Here's how the part is built. I have some questions about the finished solid (model axes, mm). A direction names the side the tool comes from. Give positions to 0.01 mm unless a question says otherwise; leave off trailing zeros. Loops run counter-clockwise (first coordinate to the right, second up) from the corner with the lowest first, then second, coordinate; pieces in that order, holes last.
Q1. We'd pull the mould along Y, two halves only. Please class faces 3 (the face through (0, 8, 4)), 4 (the face through (0, -8.5, 1)), 5 (the face through (8.5, 0, 1)), 6 (the face through (0, 2.1, 2)): +Y half, -Y half, draft (parallel to the pull), parting line (faces both ways), or undercut.
Q2. I need wall thicknesses on line 1 (Y direction, x = 3, z = 2.25); line 2 (X direction, y = -1.25, z = 1.5) (1 decimal); line 3 (X direction, y = 2, z = 2.75) (3 decimals). Which ranges of each line are inside material? Lowest first, please.
Q3. For faces 1 (the face through (0, -2.1, 2)), 2 (the face through (-8.5, 0, 1)), which set-ups out of +Z, -Z, +X, -X, +Y, -Y let a thin tool reach every point of the face, with its end or its side?
Q4. If we section it at D-D (z = 0.25): Please give me the cut outline in (x, y) (3 decimals), plus the area to 3 significant figures.
Q5. If we section it at B-B (y = 6): Please give me the cut outline in (x, z).
Q6. Will this pin go through, and if not, where does the flat tip stop? P1, Ø6.5, axis at x = 2.5, y = 2.5, coming from the -Z side.
Q7. If we section it at A-A (z = 2.25): Please give me the cut outline in (x, y) (3 decimals), plus the area to 3 significant figures.
from build123d import *
from OCP.BRepFilletAPI import BRepFilletAPI_MakeChamfer

# Parameters (mm, degrees)
SKETCH1_R           = 2.75
BOSS_EXTRUDE1_DEPTH = 4
SKETCH2_W           = 17
SKETCH2_H           = 17
BOSS_EXTRUDE2_DEPTH = 1
SKETCH3_W           = 17
SKETCH3_H           = 17
SKETCH3_W_2         = 15
SKETCH3_H_2         = 15
BOSS_EXTRUDE3_DEPTH = 6
CHAMFER1_SIZE       = 1.5
CHAMFER2_SIZE       = 4
CHAMFER2_SIZE2      = 0.5
CUT_EXTRUDE1_DEPTH  = 0.6
BOSS_EXTRUDE4_START = 0.5
SKETCH5_W           = 14.989533589
SKETCH5_H           = 15
SKETCH5_R           = 2.75
BOSS_EXTRUDE4_DEPTH = 0.5


with BuildPart() as part:
    # Sketch1 → Boss-Extrude1 (new body)
    with BuildSketch(Plane(origin=(0, 0, 0), x_dir=(0, 1, 0), z_dir=(0, 0, 1))):
        with Locations(Location((0, 0, 0), (0, 0, 270))):
            Circle(SKETCH1_R)
        Polygon((-0.7, -0.625), (-2.1, -0.625), (-2.1, 0.625), (-0.7, 0.625), (-0.7, 2.1), (0.7, 2.1), (0.7, 0.625), (2.1, 0.625), (2.1, -0.625), (0.7, -0.625), (0.7, -2.1), (-0.7, -2.1), align=None, mode=Mode.SUBTRACT)
    extrude(amount=BOSS_EXTRUDE1_DEPTH)

    # Sketch2 → Boss-Extrude2 (add)
    with BuildSketch(Plane.XY.offset(4)):
        Rectangle(SKETCH2_W, SKETCH2_H)
    extrude(amount=BOSS_EXTRUDE2_DEPTH)

    # Sketch3 → Boss-Extrude3 (add)
    with BuildSketch(Plane(origin=(0, 0, 4), x_dir=(1, 0, 0), z_dir=(0, 0, -1))):
        Rectangle(SKETCH3_W, SKETCH3_H)
        Rectangle(SKETCH3_W_2, SKETCH3_H_2, mode=Mode.SUBTRACT)
    extrude(amount=BOSS_EXTRUDE3_DEPTH)

    # Chamfer1
    chamfer1_edges = [part.edges().sort_by_distance(p)[0] for p in [
        (8.5, 0, 5),
        (0, 8.5, 5),
        (-8.5, 0, 5),
        (0, -8.5, 5),
        (-2.75, 0, 4),
        (0, -7.5, 4),
        (7.5, 0, 4),
        (-7.5, 0, 4),
        (0, 7.5, 4),
    ]]
    chamfer(chamfer1_edges, length=CHAMFER1_SIZE)

    # Chamfer2: one chamfer whose edges measure the first distance from different faces: ONE call of the kernel's chamfer builder (chamfer() names one face for all edges)
    chamfer2_edges_1 = [part.edges().sort_by_distance(p)[0] for p in [
        (-7.5, 0, -2),
    ]]
    chamfer2_side_1 = [part.faces().sort_by_distance(p)[0] for p in [
        (-7.5, 0, 0.25),
    ]]
    chamfer2_edges_2 = [part.edges().sort_by_distance(p)[0] for p in [
        (0, 7.5, -2),
    ]]
    chamfer2_side_2 = [part.faces().sort_by_distance(p)[0] for p in [
        (0, 7.5, 0.25),
    ]]
    chamfer2_edges_3 = [part.edges().sort_by_distance(p)[0] for p in [
        (0, -7.5, -2),
    ]]
    chamfer2_side_3 = [part.faces().sort_by_distance(p)[0] for p in [
        (0, -7.5, 0.25),
    ]]
    chamfer2_edges_4 = [part.edges().sort_by_distance(p)[0] for p in [
        (7.5, 0, -2),
    ]]
    chamfer2_side_4 = [part.faces().sort_by_distance(p)[0] for p in [
        (7.5, 0, 0.25),
    ]]
    chamfer2 = BRepFilletAPI_MakeChamfer(part.part.solid().wrapped)
    for e in chamfer2_edges_1:
        chamfer2.Add(CHAMFER2_SIZE, CHAMFER2_SIZE2, e.wrapped, chamfer2_side_1[0].wrapped)  # the first distance lies on this face
    for e in chamfer2_edges_2:
        chamfer2.Add(CHAMFER2_SIZE, CHAMFER2_SIZE2, e.wrapped, chamfer2_side_2[0].wrapped)  # the first distance lies on this face
    for e in chamfer2_edges_3:
        chamfer2.Add(CHAMFER2_SIZE, CHAMFER2_SIZE2, e.wrapped, chamfer2_side_3[0].wrapped)  # the first distance lies on this face
    for e in chamfer2_edges_4:
        chamfer2.Add(CHAMFER2_SIZE, CHAMFER2_SIZE2, e.wrapped, chamfer2_side_4[0].wrapped)  # the first distance lies on this face
    add(Compound.cast(chamfer2.Shape()), mode=Mode.REPLACE)

    # Sketch4 → Cut-Extrude1 (cut)
    with BuildSketch(Plane.XY.offset(5)):
        Polygon((-0.06051573, 4.249569137), (-1.192187018, 2.946103658), (-1.166609713, 1.15), (1.133856704, 1.15), (1.108279399, 2.946103658), align=None)
        Polygon((-1.166609713, 1.15), (-1.192187018, 2.946103658), (-2.751567741, 1.15), align=None)
        Polygon((-1.150233209, 0), (-1.166609713, 1.15), (-2.751567741, 1.15), (-3.75, 0), align=None)
        Polygon((1.133856704, 1.15), (-1.166609713, 1.15), (-1.150233209, 0), (1.150233209, 0), align=None)
        Polygon((2.718814732, 1.15), (1.108279399, 2.946103658), (1.133856704, 1.15), align=None)
        Polygon((2.718814732, 1.15), (1.133856704, 1.15), (1.150233209, 0), (3.75, 0), align=None)
        Polygon((1.166609713, -1.15), (-1.133856704, -1.15), (-1.08948427, -4.265945641), (1.21051573, -4.233192632), align=None)
        Polygon((1.150233209, 0), (-1.150233209, 0), (-1.133856704, -1.15), (1.166609713, -1.15), align=None)
    extrude(amount=-CUT_EXTRUDE1_DEPTH, mode=Mode.SUBTRACT)

    # Sketch5 → Boss-Extrude4 (add)
    with BuildSketch(Plane(origin=(0, 0, 4), x_dir=(1, 0, 0), z_dir=(0, 0, -1)).offset(BOSS_EXTRUDE4_START)):
        with Locations((-0.005233206, 0)):
            Rectangle(SKETCH5_W, SKETCH5_H)
        with Locations(Location((0, 0, 0), (0, 0, 180))):
            Circle(SKETCH5_R, mode=Mode.SUBTRACT)
    extrude(amount=-BOSS_EXTRUDE4_DEPTH)


solid = part.part
Check sheet entries:
1. face 3: +Y half
1. face 4: -Y half
1. face 5: draft
1. face 6: undercut
2. line 1: y = -8.5 to -7.5, 7.5 to 8.5
2. line 2: x = -8.5 to -7.6, -2.4 to -0.6, 0.6 to 2.4, 7.6 to 8.5
2. line 3: x = -8.5 to -7.25, -2.236 to -0.625, 0.625 to 2.236, 7.25 to 8.5
3. face 1: -Z
3. face 2: +Z, -Z, -X, +Y, -Y
4. outline: (-8.5, -8.5) - (8.5, -8.5) - (8.5, 8.5) - (-8.5, 8.5) - close; circle Ø5.5 at (0, 0); hole (-7.719, -7.719) - (7.719, -7.719) - (7.719, 7.719) - (-7.719, 7.719) - close; hole (-2.1, -0.7) - (-0.625, -0.7) - (-0.625, -2.1) - (0.625, -2.1) - (0.625, -0.7) - (2.1, -0.7) - (2.1, 0.7) - (0.625, 0.7) - (0.625, 2.1) - (-0.625, 2.1) - (-0.625, 0.7) - (-2.1, 0.7) - close
4. area: 65.1 mm2
5. outline: (-8.5, -2) - (-8, -2) - (-7.5, 2) - (-7.5, 2.5) - (-6.5, 3.5) - (6.5, 3.5) - (7.5, 2.5) - (7.5, 2) - (8, -2) - (8.5, -2) - (8.5, 3.5) - (7, 5) - (-7, 5) - (-8.5, 3.5) - close
6. P1: stops at z = 0
7. outline: (-8.5, -8.5) - (8.5, -8.5) - (8.5, 8.5) - (-8.5, 8.5) - close; circle Ø5.5 at (0, 0); hole (-7.5, -7.5) - (7.5, -7.5) - (7.5, 7.5) - (-7.5, 7.5) - close; hole (-2.1, -0.7) - (-0.625, -0.7) - (-0.625, -2.1) - (0.625, -2.1) - (0.625, -0.7) - (2.1, -0.7) - (2.1, 0.7) - (0.625, 0.7) - (0.625, 2.1) - (-0.625, 2.1) - (-0.625, 0.7) - (-2.1, 0.7) - close
7. area: 78.4 mm2
